Check sheet for the modelled part. Datum: model origin and axes. Units: mm. A direction names the side the tool comes from. Round coordinates to 2 decimals unless told otherwise and drop trailing zeros. Write each loop counter-clockwise with the first axis right and the second up, starting at its lowest first coordinate (ties: lowest second). Pieces come first, ordered by that corner, then holes.
Item 1: Depth check by flat-ended pin: pin 1 (5 mm diameter, centred on x = -29, y = -46, fed in from +Z); pin 2 (4 mm diameter, centred on x = 372.5, z = 350, fed in from +Y). Enter the tip coordinate at first touch or a pass-through.
Item 2: Section check C-C, the plane z = 162.5. Record the cut outline in (x, y), plus the area to 3 significant figures.
Item 3: Section check A-A, the plane y = 171.5. Record the cut outline in (x, z), plus the area to 3 significant figures.
Item 4: Release check for a two-part mould opening along X. For faces 4 (the flat face through (-265.38, -92.29, 298.6)), 5 (the flat face through (397, -228, 400)), 6 (the flat face through (26, -83, 200)), 7 (the flat face through (-417.479, -83, 197)) record: pulls with the +X half, pulls with the -X half, needs draft (parallel to the pull), parting line crosses it, or undercut.
Item 5: Section check D-D, the plane x = 34.5. Record the cut outline in (y, z).
Item 6: Section check B-B, the plane z = 278. Record the cut outline in (x, y), plus the area to 3 significant figures.
Item 7: Set-up check for faces 1 (the flat face through (-117.479, 133, 101)), 2 (the flat face through (-270, 237.262, 99)), 3 (the flat face through (334.62, -83.19, 298.6)): record each of +Z, -Z, +X, -X, +Y, -Y from which the full face is reachable in a straight line by a thin tool's end or side.
Item 8: Material ranges on line 1 along X through (y, z) = (174, 199.5); line 2 along Z through (x, y) = (-31, -247.5); line 3 along X through (y, z) = (-188, 260), recorded low to high.
from build123d import *

# Parameters (mm, degrees)
F0_W     = 900
F0_H     = 650
F1_DEPTH = 200
F3_DEPTH = 200
F5_DEPTH = 200
F6_W     = 300
F6_H     = 205.535657
F7_DEPTH = 281.52459


with BuildPart() as f1:
    # F0 (on Top) → F1 (new body)
    with BuildSketch(Plane.XY):
        with Locations((32.520793, -87.737992)):
            Rectangle(F0_W, F0_H)
    extrude(amount=F1_DEPTH)

    # F2 (on face) → F3 (join)
    with BuildSketch(Plane.XY.offset(200)):
        Polygon((-117.479207, -412.737992), (-417.479207, 237.262008), (-417.479207, -412.737992), align=None)
    extrude(amount=F3_DEPTH)

    # F4 (on face) → F5 (join)
    with BuildSketch(Plane.XY.offset(200)):
        Polygon((482.520793, -412.737992), (482.520793, 237.262008), (182.520793, -412.737992), align=None)
    extrude(amount=F5_DEPTH)

    # F6 (on face) → F7 (cut)
    with BuildSketch(Plane.XY.offset(200)):
        with Locations((32.520793, 134.49418)):
            Rectangle(F6_W, F6_H)
    extrude(amount=-F7_DEPTH, mode=Mode.SUBTRACT)


solid = f1.part
Values found:
1. pin 1: stops at z = 200
1. pin 2: stops at y = 3.22
2. outline: (-417.48, -412.74) - (482.52, -412.74) - (482.52, 237.26) - (182.52, 237.26) - (182.52, 31.73) - (-117.48, 31.73) - (-117.48, 237.26) - (-417.48, 237.26) - close
2. area: 523,000 mm2
3. outline: (-417.48, 0) - (-117.48, 0) - (-117.48, 200) - (-387.13, 200) - (-387.13, 400) - (-417.48, 400) - close; (182.52, 0) - (482.52, 0) - (482.52, 400) - (452.17, 400) - (452.17, 200) - (182.52, 200) - close
3. area: 132,000 mm2
4. face 4: undercut
4. face 5: needs draft
4. face 6: undercut
4. face 7: pulls with the -X half
5. outline: (-412.74, 0) - (31.73, 0) - (31.73, 200) - (-412.74, 200) - close
6. outline: (-417.48, -412.74) - (-117.48, -412.74) - (-417.48, 237.26) - close; (182.52, -412.74) - (482.52, -412.74) - (482.52, 237.26) - close
6. area: 195,000 mm2
7. face 1: +Z, -Z, +Y
7. face 2: +Z, -Z, +X, -X, +Y
7. face 3: +Z, +Y
8. line 1: x = -417.48 to -117.48, 182.52 to 482.52
8. line 2: z = 0 to 200
8. line 3: x = -417.48 to -221.2, 286.25 to 482.52
